Read the model definition and answer for the solid it produces. Units are mm, in the model's axes. Give positions to 0.01 mm unless a question says otherwise; leave off trailing zeros. Write each loop counter-clockwise with the first axis right and the second up, starting at its lowest first coordinate (ties: lowest second). Pieces come first, ordered by that corner, then holes. Notation, with made-up numbers: (75.25, 49.25) -> (120.25, 49.25) arc R17 cw to (120.25, 81.25) -> close; hole circle Ø2 at (60, -30.5). An arc over 180 degrees is marked (long way). Answer as CSV lines item,"result". Start each with the question number.
1. Find the intervals of material crossed by line 1 (Y direction, x = 0, z = 1.4); line 2 (X direction, y = 1.25, z = 3.95); line 3 (X direction, y = -4.5, z = 4.2), in increasing order.
2. Given pin 1 (1.5 mm diameter, centred on y = -3, z = 3.5, fed in from +X); pin 2 (1 mm diameter, centred on y = -4.5, z = 2, fed in from -X); pin 3 (2 mm diameter, centred on x = 2.5, z = 3.5, fed in from +Y), each flat-ended and moving along its own axis, determine where each tip first touches the part or whether it passes through.
3. The part is cut by section B-B, the plane y = 0. Determine the outline of the cut face in (x, z).
4. For a pull along Y with two mould halves and no side action, classify faces 1 (the flat face through (4, -4, 5)), 2 (the cylindrical face through (14.013, 0.336, 2.465)), 3 (the flat face through (8.79, -6.71, 2.46)) as pulls with the +Y half, pulls with the -Y half, needs draft (parallel to the pull), parting line crosses it, or undercut.
5. The part is cut by section D-D, the plane x = -12.5. Determine the outline of the cut face in (y, z), and give its area (3 significant figures).
6. The part is cut by section A-A, the plane z = 1.95. Determine the outline of the cut face in (x, y).
7. The part is cut by section C-C, the plane x = 0. Determine the outline of the cut face in (y, z).
Autodesk Inventor part; units mm, degrees
ref_plane "YZ Plane" through (0, 0, 0) normal (1, 0, 0) x (0, 1, 0)
ref_plane "XZ Plane" through (0, 0, 0) normal (0, 1, 0) x (-1, 0, 0)
ref_plane "XY Plane" through (0, 0, 0) normal (0, 0, 1) x (1, 0, 0)
sketch "Boceto1" plane through (0, 0, 0) normal (0, 0, 1) x (1, 0, 0)
  arc A0 (12.5, 1.55) -> (10.95, 0) centre (12.5, 0) ccw
  arc A1 (10.95, 0) -> (12.5, -1.55) centre (12.5, 0) ccw
  arc A2 (12.5, -1.55) -> (14.05, 0) centre (12.5, 0) ccw
  arc A3 (14.05, 0) -> (12.5, 1.55) centre (12.5, 0) ccw
  arc A4 (0, 4.95) -> (-4.95, 0) centre (0, 0) ccw
  arc A5 (-4.95, 0) -> (0, -4.95) centre (0, 0) ccw
  arc A6 (0, -4.95) -> (4.95, 0) centre (0, 0) ccw
  arc A7 (4.95, 0) -> (0, 4.95) centre (0, 0) ccw
  arc A8 (-12.5, 1.55) -> (-14.05, 0) centre (-12.5, 0) ccw
  arc A9 (-14.05, 0) -> (-12.5, -1.55) centre (-12.5, 0) ccw
  arc A10 (-12.5, -1.55) -> (-10.95, 0) centre (-12.5, 0) ccw
  arc A11 (-10.95, 0) -> (-12.5, 1.55) centre (-12.5, 0) ccw
  arc A12 (3.4398, 8.8017) -> (-3.4398, 8.8017) centre (0, 0) ccw
  line L0 (-3.4398, 8.8017) -> (-14.2836, 4.5639)
  arc A13 (-14.2836, 4.5639) -> (-14.2836, -4.5639) centre (-12.5, 0) ccw
  line L1 (-14.2836, -4.5639) -> (-3.4398, -8.8017)
  arc A14 (-3.4398, -8.8017) -> (3.4398, -8.8017) centre (0, 0) ccw
  line L2 (3.4398, -8.8017) -> (14.2836, -4.5639)
  arc A15 (14.2836, -4.5639) -> (14.2836, 4.5639) centre (12.5, 0) ccw
  line L3 (14.2836, 4.5639) -> (3.4398, 8.8017)
  point P0 (0, 0)
extrude "Extrusión1" add sketch "Boceto1" along normal blind 5
properties part number "fixador barra"
Results found:
1,line 1,"y = -9.45 to -4.95, 4.95 to 9.45"
1,line 2,"x = -17.24 to -13.42, -11.58 to -4.79, 4.79 to 11.58, 13.42 to 17.24"
1,line 3,"x = -14.44 to -2.06, 2.06 to 14.44"
2,pin 1,"stops at x = 16.85"
2,pin 2,"stops at x = -15.33"
2,pin 3,"stops at y = 9.33"
3,outline,"(-17.4, 0) -> (-14.05, 0) -> (-14.05, 5) -> (-17.4, 5) -> close; (-10.95, 0) -> (-4.95, 0) -> (-4.95, 5) -> (-10.95, 5) -> close; (4.95, 0) -> (10.95, 0) -> (10.95, 5) -> (4.95, 5) -> close; (14.05, 0) -> (17.4, 0) -> (17.4, 5) -> (14.05, 5) -> close"
4,face 1,"needs draft"
4,face 2,"undercut"
4,face 3,"pulls with the -Y half"
5,outline,"(-5.26, 0) -> (-1.55, 0) -> (-1.55, 5) -> (-5.26, 5) -> close; (1.55, 0) -> (5.26, 0) -> (5.26, 5) -> (1.55, 5) -> close"
5,area,"37.1 mm²"
6,outline,"(-14.28, -4.56) -> (-3.44, -8.8) arc R9.45 ccw to (3.44, -8.8) -> (14.28, -4.56) arc R4.9 ccw to (14.28, 4.56) -> (3.44, 8.8) arc R9.45 ccw to (-3.44, 8.8) -> (-14.28, 4.56) arc R4.9 ccw to start; hole circle Ø3.1 at (-12.5, 0); hole circle Ø9.9 at (0, 0); hole circle Ø3.1 at (12.5, 0)"
7,outline,"(-9.45, 0) -> (-4.95, 0) -> (-4.95, 5) -> (-9.45, 5) -> close; (4.95, 0) -> (9.45, 0) -> (9.45, 5) -> (4.95, 5) -> close"
